from build123d import *

# Parameters (mm, degrees)
F0_R     = 1.5
F1_DEPTH = 2


with BuildPart() as f1:
    # F0 (on Top) → F1 (new body)
    with BuildSketch(Plane.XY):
        with BuildLine():
            ThreePointArc((-19.197627, 1), (-18.079593, 1.5), (-16.961559, 1))
            Line((-16.961559, 1), (-15.341597, 1))
            ThreePointArc((-15.341597, 1), (-14.624629, 1.182443), (-14.082068, 1.685392))
            ThreePointArc((-14.082068, 1.685392), (-12.946894, 2.732812), (-11.447412, 3.103307))
            Line((-11.447412, 3.103307), (10.042908, 2.904272))
            ThreePointArc((10.042908, 2.904272), (12.920407, 0), (10.042908, -2.904272))
            Line((10.042908, -2.904272), (-11.447412, -3.103307))
            ThreePointArc((-11.447412, -3.103307), (-12.946894, -2.732812), (-14.082068, -1.685392))
            ThreePointArc((-14.082068, -1.685392), (-14.624629, -1.182443), (-15.341597, -1))
            Line((-15.341597, -1), (-16.961559, -1))
            ThreePointArc((-16.961559, -1), (-18.079593, -1.5), (-19.197627, -1))
            Line((-19.197627, -1), (-20.817589, -1))
            ThreePointArc((-20.817589, -1), (-21.534557, -1.182443), (-22.077118, -1.685392))
            ThreePointArc((-22.077118, -1.685392), (-23.187047, -2.719074), (-24.654291, -3.103307))
            Line((-24.654291, -3.103307), (-33.636647, -3.186497))
            ThreePointArc((-33.636647, -3.186497), (-34.524221, -3.329426), (-35.329593, -3.728912))
            Line((-35.329593, -3.728912), (-41.368579, -7.957456))
            ThreePointArc((-41.368579, -7.957456), (-42.187191, -8.361151), (-43.089309, -8.5))
            Line((-43.089309, -8.5), (-93.329593, -8.5))
            ThreePointArc((-93.329593, -8.5), (-94.0367, -8.792893), (-94.329593, -9.5))
            Line((-94.329593, -9.5), (-94.329593, -14.5))
            ThreePointArc((-94.329593, -14.5), (-94.0367, -15.207107), (-93.329593, -15.5))
            Line((-93.329593, -15.5), (-82.493807, -15.5))
            ThreePointArc((-82.493807, -15.5), (-82.111123, -15.42388), (-81.7867, -15.207107))
            Line((-81.7867, -15.207107), (-81.372486, -14.792893))
            ThreePointArc((-81.372486, -14.792893), (-81.048063, -14.57612), (-80.66538, -14.5))
            Line((-80.66538, -14.5), (-46.066168, -14.5))
            ThreePointArc((-46.066168, -14.5), (-44.261933, -14.222302), (-42.624709, -13.414912))
            Line((-42.624709, -13.414912), (-35.361857, -8.329409))
            ThreePointArc((-35.361857, -8.329409), (-34.556484, -7.929922), (-33.668911, -7.786993))
            Line((-33.668911, -7.786993), (100.835377, -6.541272))
            ThreePointArc((100.835377, -6.541272), (104.379181, -6.932181), (107.730626, -8.148393))
            Line((107.730626, -8.148393), (121.240512, -14.964079))
            ThreePointArc((121.240512, -14.964079), (122.335124, -15.364175), (123.492622, -15.5))
            Line((123.492622, -15.5), (133.670407, -15.5))
            ThreePointArc((133.670407, -15.5), (134.377514, -15.207107), (134.670407, -14.5))
            Line((134.670407, -14.5), (134.670407, -9.5))
            ThreePointArc((134.670407, -9.5), (134.377514, -8.792893), (133.670407, -8.5))
            Line((133.670407, -8.5), (124.920407, -8.5))
            ThreePointArc((124.920407, -8.5), (123.994408, -8.39134), (123.118718, -8.071263))
            Line((123.118718, -8.071263), (111.544352, -2.232039))
            ThreePointArc((111.544352, -2.232039), (110.170407, 0), (111.544352, 2.232039))
            Line((111.544352, 2.232039), (123.118718, 8.071263))
            ThreePointArc((123.118718, 8.071263), (123.994408, 8.39134), (124.920407, 8.5))
            Line((124.920407, 8.5), (133.670407, 8.5))
            ThreePointArc((133.670407, 8.5), (134.377514, 8.792893), (134.670407, 9.5))
            Line((134.670407, 9.5), (134.670407, 14.5))
            ThreePointArc((134.670407, 14.5), (134.377514, 15.207107), (133.670407, 15.5))
            Line((133.670407, 15.5), (123.492622, 15.5))
            ThreePointArc((123.492622, 15.5), (122.335124, 15.364175), (121.240512, 14.964079))
            Line((121.240512, 14.964079), (107.730626, 8.148393))
            ThreePointArc((107.730626, 8.148393), (104.379181, 6.932181), (100.835377, 6.541272))
            Line((100.835377, 6.541272), (-45.436336, 7.895978))
            ThreePointArc((-45.436336, 7.895978), (-46.986025, 8.34407), (-48.079593, 9.530001))
            Line((-48.079593, 9.530001), (-50.018206, 13.321132))
            ThreePointArc((-50.018206, 13.321132), (-51.492074, 14.912076), (-53.579593, 15.5))
            Line((-53.579593, 15.5), (-93.329593, 15.5))
            ThreePointArc((-93.329593, 15.5), (-94.0367, 15.207107), (-94.329593, 14.5))
            Line((-94.329593, 14.5), (-94.329593, 9.5))
            ThreePointArc((-94.329593, 9.5), (-94.0367, 8.792893), (-93.329593, 8.5))
            Line((-93.329593, 8.5), (-73.90802, 8.5))
            ThreePointArc((-73.90802, 8.5), (-73.525337, 8.57612), (-73.200914, 8.792893))
            Line((-73.200914, 8.792893), (-72.0367, 9.957107))
            ThreePointArc((-72.0367, 9.957107), (-71.712277, 10.17388), (-71.329593, 10.25))
            Line((-71.329593, 10.25), (-54.49502, 10.25))
            ThreePointArc((-54.49502, 10.25), (-52.929381, 9.809057), (-51.82398, 8.615849))
            Line((-51.82398, 8.615849), (-50.223606, 5.486174))
            ThreePointArc((-50.223606, 5.486174), (-48.765515, 3.904933), (-46.699263, 3.307478))
            Line((-46.699263, 3.307478), (-24.654291, 3.103307))
            ThreePointArc((-24.654291, 3.103307), (-23.187047, 2.719074), (-22.077118, 1.685392))
            ThreePointArc((-22.077118, 1.685392), (-21.534557, 1.182443), (-20.817589, 1))
            Line((-20.817589, 1), (-19.197627, 1))
        make_face()
        with Locations((-91.079593, -12)):
            Circle(F0_R, mode=Mode.SUBTRACT)
        with Locations((-85.079593, -12)):
            Circle(F0_R, mode=Mode.SUBTRACT)
        with Locations((125.420407, -12)):
            Circle(F0_R, mode=Mode.SUBTRACT)
        with Locations((131.420407, -12)):
            Circle(F0_R, mode=Mode.SUBTRACT)
        with BuildLine():
            ThreePointArc((73.626358, 2.315394), (75.920407, 0), (73.626358, -2.315394))
            Line((73.626358, -2.315394), (30.658988, -2.713339))
            ThreePointArc((30.658988, -2.713339), (27.920407, 2e-06), (30.658992, 2.713339))
            Line((30.658992, 2.713339), (73.626358, 2.315394))
        make_face(mode=Mode.SUBTRACT)
        with Locations((-91.079593, 12)):
            Circle(F0_R, mode=Mode.SUBTRACT)
        with Locations((-85.079593, 12)):
            Circle(F0_R, mode=Mode.SUBTRACT)
        with Locations((96.420407, 0)):
            Circle(F0_R, mode=Mode.SUBTRACT)
        with Locations((125.420407, 12)):
            Circle(F0_R, mode=Mode.SUBTRACT)
        with Locations((131.420407, 12)):
            Circle(F0_R, mode=Mode.SUBTRACT)
    extrude(amount=F1_DEPTH)


solid = f1.part
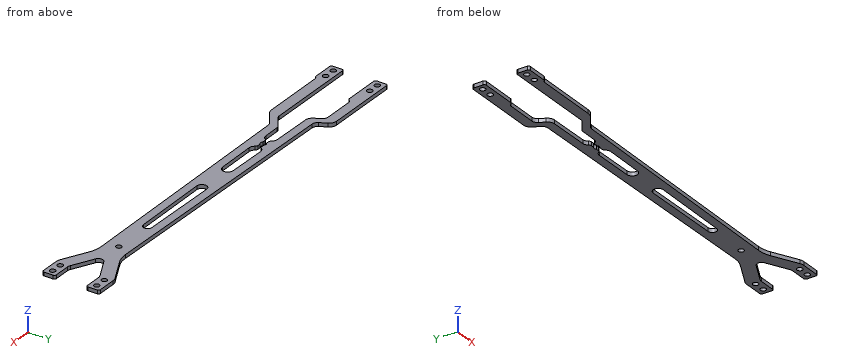
Here's how the part is built. I have some questions about the finished solid (model axes, mm). Coordinates: 2 decimals unless noted, no trailing zeros. Write each loop counter-clockwise with the first axis right and the second up, starting at its lowest first coordinate (ties: lowest second). Pieces come first, ordered by that corner, then holes.
Item 1: I want a section at C-C on x = 17. Write out the boundary of the cut face in (y, z), and give its area (3 significant figures).
Item 2: If I drill on line 1 (Y direction, x = -58.5, z = 0.45); line 2 (X direction, y = 11.5, z = 1.4); line 3 (X direction, y = 0.5, z = 0.75), over which ranges is the centre line in solid material (lowest first)?
Item 3: I want a section at A-A on z = 1.1. Count the separate pieces of the cut face and the enclosed holes in it, and give its area (3 significant figures).
Item 4: I want a section at B-B on x = 104. Write out the boundary of the cut face in (y, z), and give its area (3 significant figures).
Item 5: Will these pins go through, and if not, where does the flat tip stop? pin 1 (1 mm diameter, centred on y = -2, z = 0.5, fed in from -X); pin 2 (1 mm diameter, centred on x = -65.5, z = 1, fed in from -Y); pin 3 (0.8 mm diameter, centred on x = -19.5, z = 1, fed in from -Y).
Findings below:
1. outline: (-7.32, 0) - (7.32, 0) - (7.32, 2) - (-7.32, 2) - close
1. area: 29.3 mm2
2. line 1: y = -14.5 to -8.5, 10.25 to 15.5
2. line 2: x = -94.33 to -92.49, -89.67 to -86.49, -83.67 to -49.09, 114.37 to 124.01, 126.83 to 130.01, 132.83 to 134.67
2. line 3: x = 12.88 to 27.97, 75.87 to 95.01, 97.83 to 110.22
3. separate pieces: 1
3. enclosed holes: 10
3. area: 2,610 mm2
4. outline: (-6.85, 0) - (6.85, 0) - (6.85, 2) - (-6.85, 2) - close
4. area: 27.4 mm2
5. pin 1: stops at x = -22.84
5. pin 2: stops at y = -14.5
5. pin 3: stops at y = -7.66
